Read the model definition and answer for the solid it produces. Units are mm, in the model's axes. Face numbers are marked on the shaded views. A direction names the side the tool comes from. Coordinates: 2 decimals unless noted, no trailing zeros. Write each loop counter-clockwise with the first axis right and the second up, starting at its lowest first coordinate (ties: lowest second). Pieces come first, ordered by that corner, then holes. Notation, with made-up numbers: (73, 40.5) - (81, 40.5) arc R30 cw to (81, 67.5) - close; hole circle Ø1 at (-15.75, 33.25). An arc over 180 degrees is marked (long way). Return JSON: item names as keys, results as strings.
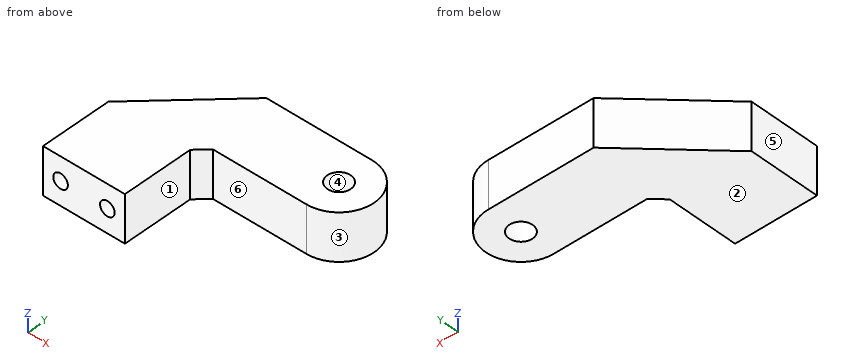
```python
from build123d import *

# Parameters (mm, degrees)
ESQUISSE1_W             = 14
ESQUISSE1_H             = 26
BOSS_EXTRU_1_DEPTH      = 8
ESQUISSE3_R             = 1.25
ENL_V_MAT_EXTRU_1_DEPTH = 10
ESQUISSE4_W             = 24
ESQUISSE4_H             = 12
BOSS_EXTRU_2_DEPTH      = 8
ESQUISSE5_R             = 2
ENL_V_MAT_EXTRU_2_DEPTH = 42.243181255
CHANFREIN1_SIZE         = 14
ENL_V_MAT_EXTRU_3_DEPTH = 42.243181255
CHANFREIN2_SIZE         = 2


with BuildPart() as part:
    # Esquisse1 → Boss.-Extru.1 (new body)
    with BuildSketch(Plane.XY):
        with Locations((0, 13)):
            Rectangle(ESQUISSE1_W, ESQUISSE1_H)
    extrude(amount=BOSS_EXTRU_1_DEPTH)

    # Esquisse3 → Enlèv. mat.-Extru.1 (cut)
    with BuildSketch(Plane(origin=(0, 0, 0), x_dir=(-1, 0, 0), z_dir=(0, -1, 0))):
        with Locations(Location((4, -4, 0), (0, 0, 180))):
            Circle(ESQUISSE3_R)
        with Locations((-4, -4)):
            Circle(ESQUISSE3_R)
    extrude(amount=-ENL_V_MAT_EXTRU_1_DEPTH, mode=Mode.SUBTRACT)

    # Esquisse4 → Boss.-Extru.2 (add)
    with BuildSketch(Plane.XY.offset(8)):
        with Locations((19, 20)):
            Rectangle(ESQUISSE4_W, ESQUISSE4_H)
    extrude(amount=-BOSS_EXTRU_2_DEPTH)

    # Esquisse5 → Enlèv. mat.-Extru.2 (cut, through all)
    with BuildSketch(Plane.XY.offset(8)):
        with Locations((25, 20)):
            Circle(ESQUISSE5_R)
    extrude(amount=-ENL_V_MAT_EXTRU_2_DEPTH, mode=Mode.SUBTRACT)

    # Chanfrein1
    chanfrein1_edges = [part.edges().sort_by_distance(p)[0] for p in [
        (-7, 26, 4),
    ]]
    chamfer(chanfrein1_edges, length=CHANFREIN1_SIZE)

    # Esquisse6 → Enlèv. mat.-Extru.3 (cut, through all)
    with BuildSketch(Plane.XY.offset(8)):
        with BuildLine():
            Line((25, 26), (32, 26))
            Line((32, 26), (32, 14))
            Line((32, 14), (25, 14))
            ThreePointArc((25, 14), (31, 20), (25, 26))
        make_face()
    extrude(amount=-ENL_V_MAT_EXTRU_3_DEPTH, mode=Mode.SUBTRACT)

    # Chanfrein2
    chanfrein2_edges = [part.edges().sort_by_distance(p)[0] for p in [
        (7, 14, 4),
    ]]
    chamfer(chanfrein2_edges, length=CHANFREIN2_SIZE)


solid = part.part
```
(1) Which of the six approach directions +Z, -Z, +X, -X, +Y, -Y give full straight-line access (tool end or side, diameter ignored) to the marked faces 1 and 2?
Answer:
{"face 1": "+Z, -Z, +X, -Y", "face 2": "-Z, +X, -X, +Y, -Y"}
(2) A cutting plane is placed at D-D (z = 4). Determine the outline of the cut face in (x, y), and give its area (3 significant figures).
Answer:
{"outline": "(-7, 0) - (-5.25, 0) - (-5.25, 10) - (-2.75, 10) - (-2.75, 0) - (2.75, 0) - (2.75, 10) - (5.25, 10) - (5.25, 0) - (7, 0) - (7, 12) - (9, 14) - (25, 14) arc R6 ccw to (25, 26) - (7, 26) - (-7, 12) - close; hole circle Ø4 at (25, 20)", "area": "478 mm²"}
(3) A cutting plane is placed at B-B (x = -4). Determine the outline of the cut face in (y, z), and give its area (3 significant figures).
Answer:
{"outline": "(0, 0) - (15, 0) - (15, 8) - (0, 8) - (0, 5.25) - (10, 5.25) - (10, 2.75) - (0, 2.75) - close", "area": "95.0 mm²"}
(4) Flat-ended cylindrical pins translate along their axes: P1, Ø1.5, axis at y = 18, z = 4.5, coming from the -X side; P2, Ø1.5, axis at y = 16, z = 5.5, coming from the -X side; P3, Ø4, axis at x = 16.5, z = 5.5, coming from the -Y side; P4, Ø4, axis at x = 14, y = 10.5, coming from the -Z side. Find the tip coordinate at first contact, or state that the pin passes through.
Answer:
{"P1": "x = -1.75", "P2": "x = -3.75", "P3": "y = 14", "P4": "through"}
(5) A cutting plane is placed at C-C (y = 4.25). Determine the outline of the cut face in (x, z).
Answer:
{"outline": "(-7, 0) - (7, 0) - (7, 8) - (-7, 8) - close; hole circle Ø2.5 at (-4, 4); hole circle Ø2.5 at (4, 4)"}
(6) A cutting plane is placed at A-A (z = 7.5). Determine the outline of the cut face in (x, y), and give its area (3 significant figures).
Answer:
{"outline": "(-7, 0) - (7, 0) - (7, 12) - (9, 14) - (25, 14) arc R6 ccw to (25, 26) - (7, 26) - (-7, 12) - close; hole circle Ø4 at (25, 20)", "area": "528 mm²"}
(7) Determine the mould class of the marked faces 3, 4, 5 and 6 for opening direction Y: +Y half, -Y half, draft (parallel to the pull), parting line (faces both ways), or undercut.
Answer:
{"face 3": "parting line", "face 4": "undercut", "face 5": "draft", "face 6": "-Y half"}
(8) Straight lines are drawn through the part: line 1 (Z direction, x = 4, y = 7); line 2 (Y direction, x = 25, z = 4); line 3 (X direction, y = 7.25, z = 0.75). For each, find the intervals that lie inside material, in ascending order. Write a range as from..to.
Answer:
{"line 1": "0..2.75, 5.25..8", "line 2": "14..18, 22..26", "line 3": "-7..7"}
